from build123d import *

# Parameters (mm, degrees)
F1_DEPTH = 13.462
F2_DEPTH = 7.874
F3_DEPTH = 12.7
F0_W     = 6.35
F0_H     = 28.575
F4_DEPTH = 7.874
F5_W     = 6.35
F5_H     = 28.575
F6_DEPTH = 4.826


with BuildPart() as f1:
    # F0 (on Front) → F1 (new body, symmetric)
    with BuildSketch(Plane.XZ):
        Polygon((-67.056, -15.875), (0, -15.875), (0, 15.875), (-67.056, 15.875), (-73.406, 15.875), (-73.406, -15.875), align=None)
    extrude(amount=F1_DEPTH, both=True)

    # F0 (on Front) → F2 (join, symmetric)
    with BuildSketch(Plane.XZ):
        Polygon((-3.81, -26.924), (13.716, -26.924), (2.667, -15.875), (0, -15.875), (-67.056, -15.875), (-67.056, -44.45), (-3.81, -44.45), align=None)
        with BuildLine():
            ThreePointArc((-19.304, -24.638), (-13.716, -30.226), (-19.304, -35.814))
            Line((-19.304, -35.814), (-43.18, -35.814))
            ThreePointArc((-43.18, -35.814), (-48.768, -30.226), (-43.18, -24.638))
            Line((-43.18, -24.638), (-19.304, -24.638))
        make_face(mode=Mode.SUBTRACT)
        Polygon((-67.056, 15.875), (0, 15.875), (2.667, 15.875), (13.716, 26.924), (-3.81, 26.924), (-3.81, 44.45), (-67.056, 44.45), align=None)
        with BuildLine():
            ThreePointArc((-19.304, 35.814), (-13.716, 30.226), (-19.304, 24.638))
            Line((-19.304, 24.638), (-43.18, 24.638))
            ThreePointArc((-43.18, 24.638), (-48.768, 30.226), (-43.18, 35.814))
            Line((-43.18, 35.814), (-19.304, 35.814))
        make_face(mode=Mode.SUBTRACT)
    extrude(amount=F2_DEPTH, both=True)

    # F0 (on Front) → F3 (join, symmetric)
    with BuildSketch(Plane.XZ):
        Polygon((-3.81, 26.924), (13.716, 26.924), (31.242, 44.45), (-3.81, 44.45), align=None)
        Polygon((-3.81, -44.45), (31.242, -44.45), (13.716, -26.924), (-3.81, -26.924), align=None)
    extrude(amount=F3_DEPTH, both=True)

    # F0 (on Front) → F4 (join, symmetric)
    with BuildSketch(Plane.XZ):
        with Locations((-70.231, 30.1625)):
            Rectangle(F0_W, F0_H)
        with Locations((-70.231, -30.1625)):
            Rectangle(F0_W, F0_H)
    extrude(amount=F4_DEPTH, both=True)

    # F5 (on face) → F6 (cut)
    with BuildSketch(Plane.XZ.offset(7.874)):
        with Locations((-70.231, 30.1625)):
            Rectangle(F5_W, F5_H)
        with Locations((-70.231, -30.1625)):
            Rectangle(F5_W, F5_H)
    extrude(amount=-F6_DEPTH, mode=Mode.SUBTRACT)


solid = f1.part
Work out the finished part from the listing and answer in its coordinate system (mm). A direction names the side the tool comes from. Round coordinates to 2 decimals unless told otherwise and drop trailing zeros. Write each loop counter-clockwise with the first axis right and the second up, starting at its lowest first coordinate (ties: lowest second). Pieces come first, ordered by that corner, then holes. Notation, with made-up numbers: M -22.75,59 L 33.25,59 A21 ccw 33.25,68 Z; hole C -23,68.5 d2. An arc over 180 degrees is marked long. Use a Markdown table: item, result.
1) Which of the six approach directions +Z, -Z, +X, -X, +Y, -Y give full straight-line access (tool end or side, diameter ignored) to faces 1 (the face through (10, 12.7, 36)), 2 (the face through (-3.81, 10, -36)), 3 (the face through (19.93, -0.18, 33.14)), 4 (the face through (-48.767, -0.11, 30.103))?
Taken from the geometry:
| item | result |
|---|---|
| face 1 | +Z, +X, -X, +Y |
| face 2 | -Z, -X, +Y |
| face 3 | +X, +Y, -Y |
| face 4 | +Y, -Y |
2) The part is cut by section C-C on y = -5. Give the vertices of the cut face in (x, z) (3 decimals).
Taken from the geometry:
| item | result |
|---|---|
| outline | M -73.406,-15.875 L -67.056,-15.875 L -67.056,-44.45 L 31.242,-44.45 L 2.667,-15.875 L 0,-15.875 L 0,15.875 L 2.667,15.875 L 31.242,44.45 L -67.056,44.45 L -67.056,15.875 L -73.406,15.875 Z; hole M -43.18,-35.814 L -19.304,-35.814 A5.588 ccw -19.304,-24.638 L -43.18,-24.638 A5.588 ccw Z; hole M -43.18,24.638 L -19.304,24.638 A5.588 ccw -19.304,35.814 L -43.18,35.814 A5.588 ccw Z |
3) The part is cut by section B-B on x = -23. Give the vertices of the cut face in (y, z) (3 decimals), plus the area to 3 significant figures.
Taken from the geometry:
| item | result |
|---|---|
| outline | M -13.462,-15.875 L -7.874,-15.875 L -7.874,-24.638 L 7.874,-24.638 L 7.874,-15.875 L 13.462,-15.875 L 13.462,15.875 L 7.874,15.875 L 7.874,24.638 L -7.874,24.638 L -7.874,15.875 L -13.462,15.875 Z; M -7.874,-44.45 L 7.874,-44.45 L 7.874,-35.814 L -7.874,-35.814 Z; M -7.874,35.814 L 7.874,35.814 L 7.874,44.45 L -7.874,44.45 Z |
| area | 1,400 mm2 |
4) The part is cut by section A-A on y = 10. Give the vertices of the cut face in (x, z) (3 decimals), plus the area to 3 significant figures.
Taken from the geometry:
| item | result |
|---|---|
| outline | M -73.406,-15.875 L 0,-15.875 L 0,15.875 L -73.406,15.875 Z; M -3.81,-44.45 L 31.242,-44.45 L 13.716,-26.924 L -3.81,-26.924 Z; M -3.81,26.924 L 13.716,26.924 L 31.242,44.45 L -3.81,44.45 Z |
| area | 3,250 mm2 |
5) Consider line 1 (Z direction, x = -25, y = 1.5); line 2 (Z direction, x = -18.5, y = 2.25); line 3 (Z direction, x = -39.5, y = -10) (3 decimals). Determine where each line is inside the solid, lowest interval first. Write a range as [from, to].
Taken from the geometry:
| item | result |
|---|---|
| line 1 | z = [-44.45, -35.81], [-24.64, 24.64], [35.81, 44.45] |
| line 2 | z = [-44.45, -35.76], [-24.7, 24.7], [35.76, 44.45] |
| line 3 | z = [-15.875, 15.875] |
6) The part is cut by section D-D on x = -52. Give the vertices of the cut face in (y, z) (3 decimals).
Taken from the geometry:
| item | result |
|---|---|
| outline | M -13.462,-15.875 L -7.874,-15.875 L -7.874,-44.45 L 7.874,-44.45 L 7.874,-15.875 L 13.462,-15.875 L 13.462,15.875 L 7.874,15.875 L 7.874,44.45 L -7.874,44.45 L -7.874,15.875 L -13.462,15.875 Z |
7) Flat-ended cylindrical pins translate along their axes: pin 1 (1 mm diameter, centred on x = -12.5, y = 11, fed in from +Z) (3 decimals); pin 2 (23 mm diameter, centred on x = -46.5, z = -24, fed in from -Y); pin 3 (19.5 mm diameter, centred on x = 9, z = -33, fed in from +Y); pin 4 (8.5 mm diameter, centred on x = -16, z = 25.5, fed in from -Y). Find the tip coordinate at first contact, or state that the pin passes through.
Taken from the geometry:
| item | result |
|---|---|
| pin 1 | stops at z = 15.875 |
| pin 2 | stops at y = -13.46 |
| pin 3 | stops at y = 12.7 |
| pin 4 | stops at y = -7.87 |
8) Determine the mould class of faces 5 (the face through (5, 10, -26.924)), 6 (the face through (10, 12.7, -36)), 7 (the face through (-31, 0, 35.814)), 8 (the face through (-10, 0, 44.45)) for opening direction Z: pulls with the +Z half, pulls with the -Z half, needs draft (parallel to the pull), parting line crosses it, or undercut.
Taken from the geometry:
| item | result |
|---|---|
| face 5 | undercut |
| face 6 | needs draft |
| face 7 | undercut |
| face 8 | pulls with the +Z half |
